Source: CAD feature listing. Evaluate the final solid. Frame: model axes, mm. A direction names the side the tool comes from. Coordinates: 2 decimals unless noted, no trailing zeros. Write each loop counter-clockwise with the first axis right and the second up, starting at its lowest first coordinate (ties: lowest second). Pieces come first, ordered by that corner, then holes. Notation, with made-up numbers: M -8.75,56 L 31.25,56 A31 ccw 31.25,94 Z; hole C 16,81 d9. An arc over 180 degrees is marked long. One line per item, written item: value. Start each with the question number.
Item 1: Cut plane A-A, the plane z = 37.5. Output: boundary loops of the cut face in (x, y), then the cut area to 3 significant figures.
Item 2: Cut plane B-B, the plane x = 12.5. Output: boundary loops of the cut face in (y, z), then the cut area to 3 significant figures.
Item 3: Ray query, L1, parallel to X at y = 0.35, z = -12.5; L2, parallel to X at y = 0.8, z = 37.5; L3, parallel to Z at x = 11.5, y = 0.5. Return the intervals inside material, ascending. Write a range as from..to.
Item 4: Mould query, pull axis X, two halves, no side actions, for faces 3 (the cylindrical face through (12.5, 0.8, -19.5)), 4 (the cylindrical face through (-16.93, 0.81, -51.4)), 5 (the cylindrical face through (16.9, 0.81, 51.43)). Classes: released by +X, released by -X, zero draft, split by the parting line, or undercut.
Item 5: Set-up query: faces 1 (the cylindrical face through (-16.93, 0.81, 51.4)), 2 (the cylindrical face through (12.5, 0.8, -5.5)). Return all of +Z, -Z, +X, -X, +Y, -Y with unobstructed straight access to the full face (end or side cutting, diameter ignored); none if empty.
Item 6: Cut plane D-D, the plane y = 0.4. Output: boundary loops of the cut face in (x, z).
Item 7: Cut plane C-C, the plane x = 0. Output: boundary loops of the cut face in (y, z), then the cut area to 3 significant figures.
```python
from build123d import *

# Parameters (mm, degrees)
SKETCH_1_W          = 35
SKETCH_1_H          = 104
EXTRUDE_1_DEPTH     = 1.6
SKETCH_3_R          = 2
CUT_EXTRUDE_1_DEPTH = 55.88906995
CUT_EXTRUDE_2_DEPTH = 55.88906995
FILLET_1_R          = 2


with BuildPart() as part:
    # 草图1 → 凸台-拉伸1 (new body)
    with BuildSketch(Plane(origin=(0, 0, 0), x_dir=(1, 0, 0), z_dir=(0, 1, 0))):
        Rectangle(SKETCH_1_W, SKETCH_1_H)
    extrude(amount=EXTRUDE_1_DEPTH)

    # 草图3 → 切除-拉伸1 (cut, through all)
    with BuildSketch(Plane(origin=(0, 1.6, 0), x_dir=(1, 0, 0), z_dir=(0, 1, 0))):
        with Locations(Location((0, 12.5, 0), (0, 0, 270))):
            Circle(SKETCH_3_R)
        with Locations(Location((0, -37.5, 0), (0, 0, 270))):
            Circle(SKETCH_3_R)
    extrude(amount=-CUT_EXTRUDE_1_DEPTH, mode=Mode.SUBTRACT)

    # 草图4 → 切除-拉伸2 (cut, through all)
    with BuildSketch(Plane(origin=(0, 1.6, 0), x_dir=(1, 0, 0), z_dir=(0, 1, 0))):
        with BuildLine():
            Line((10.5, 7.5), (10.5, 17.5))
            ThreePointArc((10.5, 17.5), (12.5, 19.5), (14.5, 17.5))
            Line((14.5, 17.5), (14.5, 7.5))
            ThreePointArc((14.5, 7.5), (12.5, 5.5), (10.5, 7.5))
        make_face()
        with BuildLine():
            Line((-10.5, 7.5), (-10.5, 17.5))
            ThreePointArc((-10.5, 17.5), (-12.5, 19.5), (-14.5, 17.5))
            Line((-14.5, 17.5), (-14.5, 7.5))
            ThreePointArc((-14.5, 7.5), (-12.5, 5.5), (-10.5, 7.5))
        make_face()
    extrude(amount=-CUT_EXTRUDE_2_DEPTH, mode=Mode.SUBTRACT)

    # 圆角1
    fillet_1_edges = [part.edges().sort_by_distance(p)[0] for p in [
        (17.5, 0.8, 52),
        (-17.5, 0.8, 52),
        (-17.5, 0.8, -52),
        (17.5, 0.8, -52),
    ]]
    fillet(fillet_1_edges, radius=FILLET_1_R)


solid = part.part
```
From the geometry:
1. outline: M -17.5,0 L -2,0 L -2,1.6 L -17.5,1.6 Z; M 2,0 L 17.5,0 L 17.5,1.6 L 2,1.6 Z
1. area: 49.6 mm²
2. outline: M 0,-52 L 1.6,-52 L 1.6,-19.5 L 0,-19.5 Z; M 0,-5.5 L 1.6,-5.5 L 1.6,52 L 0,52 Z
2. area: 144 mm²
3. L1: x = -17.5..-14.5, -10.5..-2, 2..10.5, 14.5..17.5
3. L2: x = -17.5..-2, 2..17.5
3. L3: z = -52..-19.23, -5.77..52
4. face 3: undercut
4. face 4: released by -X
4. face 5: released by +X
5. face 1: +Z, -X, +Y, -Y
5. face 2: +Y, -Y
6. outline: M -17.5,-50 A2 ccw -15.5,-52 L 15.5,-52 A2 ccw 17.5,-50 L 17.5,50 A2 ccw 15.5,52 L -15.5,52 A2 ccw -17.5,50 Z; hole M -14.5,-17.5 A2 ccw -10.5,-17.5 L -10.5,-7.5 A2 ccw -14.5,-7.5 Z; hole C 0,-12.5 d4; hole C 0,37.5 d4; hole M 10.5,-17.5 A2 ccw 14.5,-17.5 L 14.5,-7.5 A2 ccw 10.5,-7.5 Z
7. outline: M 0,-52 L 1.6,-52 L 1.6,-14.5 L 0,-14.5 Z; M 0,-10.5 L 1.6,-10.5 L 1.6,35.5 L 0,35.5 Z; M 0,39.5 L 1.6,39.5 L 1.6,52 L 0,52 Z
7. area: 154 mm²
